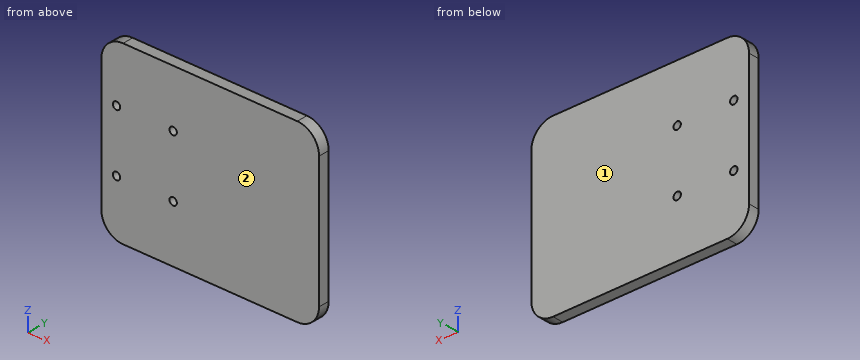
from build123d import *

# Parameters (mm, degrees)
SKETCH1_W            = 100
SKETCH1_H            = 80
BOSS_EXTRUDE1_DEPTH  = 5
M3_CLEARANCE_HOLE1_D = 3.4
FILLET1_R            = 10


with BuildPart() as part:
    # Sketch1 → Boss-Extrude1 (new body)
    with BuildSketch(Plane(origin=(0, 0, 0), x_dir=(1, 0, 0), z_dir=(0, 1, 0))):
        with Locations((30, 0)):
            Rectangle(SKETCH1_W, SKETCH1_H)
    extrude(amount=-BOSS_EXTRUDE1_DEPTH)

    # M3 Clearance Hole1 (through all)
    with Locations(Plane(origin=(-13, 0, -14), x_dir=(0, 0, 1), z_dir=(0, 1, 0))):
        with Locations((0, 0), (0, 26), (28, 26), (28, 0)):
            Hole(M3_CLEARANCE_HOLE1_D / 2)

    # Fillet1
    fillet1_edges = [part.edges().sort_by_distance(p)[0] for p in [
        (-20, -2.5, -40),
        (80, -2.5, -40),
        (80, -2.5, 40),
        (-20, -2.5, 40),
    ]]
    fillet(fillet1_edges, radius=FILLET1_R)


solid = part.part
The listing builds one solid part. Answer for the finished solid, in the listing's coordinates (mm). Face numbers are marked on the shaded views. Give positions to 0.01 mm unless a question says otherwise; leave off trailing zeros. Loops run counter-clockwise (first coordinate to the right, second up) from the corner with the lowest first, then second, coordinate; pieces in that order, holes last.
Item 1: Determine the mould class of the marked faces 1 and 2 for opening direction Y: +Y half, -Y half, draft (parallel to the pull), parting line (faces both ways), or undercut.
Derived:
face 1: +Y half
face 2: -Y half
Item 2: A cutting plane is placed at B-B (z = 14). Give the vertices of the cut face in (x, y).
Derived:
outline: (-20, -5) - (-14.7, -5) - (-14.7, 0) - (-20, 0) - close; (-11.3, -5) - (11.3, -5) - (11.3, 0) - (-11.3, 0) - close; (14.7, -5) - (80, -5) - (80, 0) - (14.7, 0) - close
Item 3: Find the intervals of material crossed by line 1 along X through (y, z) = (-3.1, 14); line 2 along X through (y, z) = (-3, -32); line 3 along Z through (x, y) = (72, -1.2), in increasing order.
Derived:
line 1: x = -20 to -14.7, -11.3 to 11.3, 14.7 to 80
line 2: x = -19.8 to 79.8
line 3: z = -39.8 to 39.8
Item 4: A cutting plane is placed at A-A (y = -2.75). Give the vertices of the cut face in (x, z), then the cut area to 3 significant figures.
Derived:
outline: (-20, -30) arc R10 ccw to (-10, -40) - (70, -40) arc R10 ccw to (80, -30) - (80, 30) arc R10 ccw to (70, 40) - (-10, 40) arc R10 ccw to (-20, 30) - close; hole circle Ø3.4 at (-13, -14); hole circle Ø3.4 at (-13, 14); hole circle Ø3.4 at (13, -14); hole circle Ø3.4 at (13, 14)
area: 7,880 mm2
Item 5: A cutting plane is placed at C-C (x = -13). Give the vertices of the cut face in (y, z).
Derived:
outline: (-5, -39.54) - (0, -39.54) - (0, -15.7) - (-5, -15.7) - close; (-5, -12.3) - (0, -12.3) - (0, 12.3) - (-5, 12.3) - close; (-5, 15.7) - (0, 15.7) - (0, 39.54) - (-5, 39.54) - close
Item 6: This flat-tipped pin is pushed along its axis until it touches: pin 1 Ø3 at (x, z) = (-13, 14) entering from -Y. Where does it stop, or does it pass through?
Derived:
pin 1: passes through
